Here's the drawing with two shaded views (mm, measured from the low corner). I have some questions. A direction names the side the tool comes from. Coordinates: 2 decimals unless noted, no trailing zeros. Write each loop counter-clockwise with the first axis right and the second up, starting at its lowest first coordinate (ties: lowest second). Pieces come first, ordered by that corner, then holes. Notation, with made-up numbers: (72, 25.5) -> (122, 25.5) arc R14 ccw to (122, 30.5) -> close; hole circle Ø1 at (-10, -8). An arc over 180 degrees is marked (long way). Use one line per item in the form item = value.
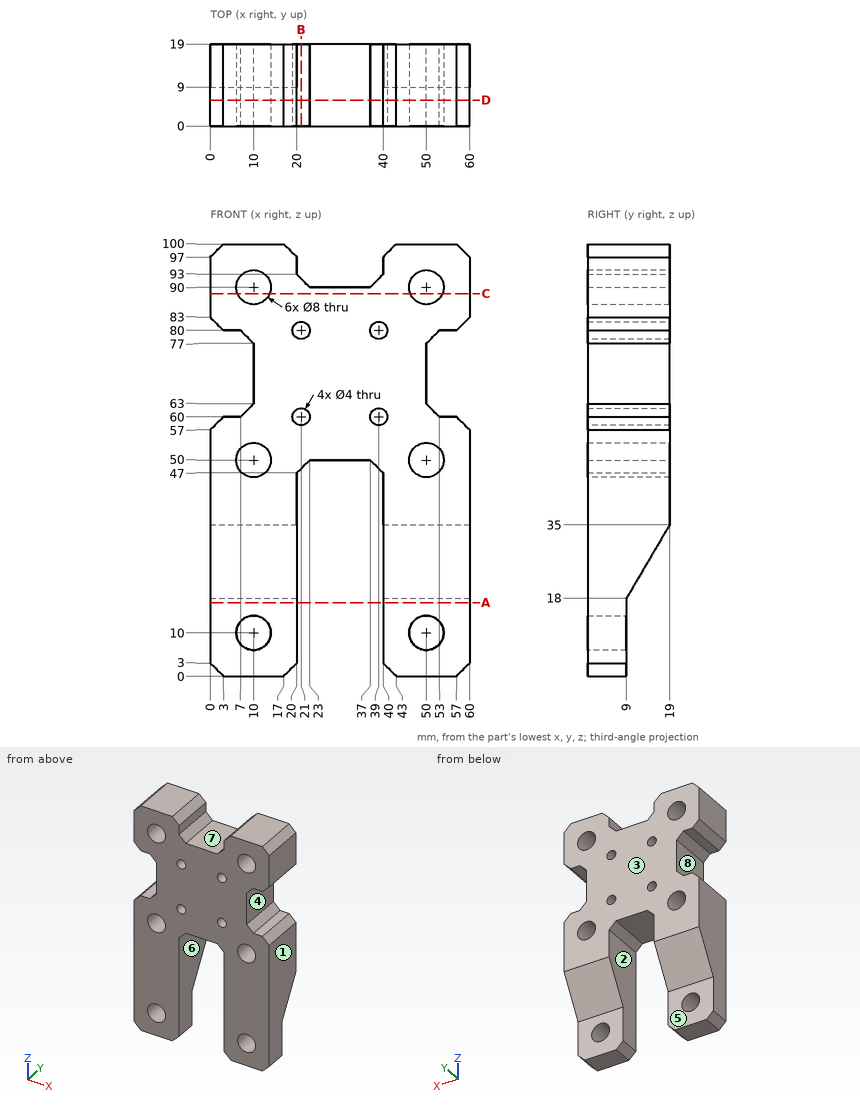
Q1. Suppose I cut it at A-A (z = 17). Write out the boundary of the cut face in (x, y), then the cut area to 3 significant figures.
Return value:
outline = (0, 0) -> (20, 0) -> (20, 9) -> (0, 9) -> close; (40, 0) -> (60, 0) -> (60, 9) -> (40, 9) -> close
area = 360 mm2
Q2. Suppose I cut it at B-B (x = 21). Write out the boundary of the cut face in (y, z).
Return value:
outline = (0, 48) -> (19, 48) -> (19, 58) -> (0, 58) -> close; (0, 62) -> (19, 62) -> (19, 78) -> (0, 78) -> close; (0, 82) -> (19, 82) -> (19, 92) -> (0, 92) -> close
Q3. If I drill on line 1 (X direction, y = 1.25, z = 31); line 2 (X direction, y = 2.25, z = 10); line 3 (X direction, y = 6.25, z = 86.5), over which ranges is the centre line in solid material (lowest first)? Write a range as from..to.
Return value:
line_1 = 0..20, 40..60
line_2 = 0..6, 14..20, 40..46, 54..60
line_3 = 0..8.06, 11.94..48.06, 51.94..60
Q4. Will these pins go through, and if not, where does the flat tip stop? pin 1 (8 mm diameter, centred on x = 37.5, z = 51, fed in from -Y); pin 2 (4 mm diameter, centred on x = 20, y = 5.5, fed in from -Z); pin 3 (11 mm diameter, centred on y = 9.5, z = 73, fed in from -X); pin 4 (5.5 mm diameter, centred on x = 8, z = 7, fed in from +Y).
Return value:
pin_1 = 0
pin_2 = 1
pin_3 = 8.5
pin_4 = 9
Q5. For the marked faces 4, 5, 6, 7 and 8, which set-ups out of +Z, -Z, +X, -X, +Y, -Y let a thin tool reach every point of the face, with its end or its side?
Return value:
face_4 = +X, +Y, -Y
face_5 = -Z, +X, -X, +Y
face_6 = -Z, +Y, -Y
face_7 = +Z, +Y, -Y
face_8 = -X, +Y, -Y
Q6. Suppose I cut it at D-D (y = 6). Give the number of separate pieces and of enclosed holes in the cut face, then the cut area to 3 significant figures.
Return value:
separate_pieces = 1
enclosed_holes = 10
area = 4,030 mm2
Q7. Suppose I cut it at C-C (z = 88.5). Write out the boundary of the cut face in (x, y).
Return value:
outline = (0, 0) -> (6.29, 0) -> (6.29, 19) -> (0, 19) -> close; (13.71, 0) -> (46.29, 0) -> (46.29, 19) -> (13.71, 19) -> close; (53.71, 0) -> (60, 0) -> (60, 19) -> (53.71, 19) -> close
Q8. Thinking about a two-plate mould opening in X: for the marked faces 1, 2 and 3, which applies, released by +X, released by -X, zero draft, split by the parting line, or undercut?
Return value:
face_1 = released by +X
face_2 = undercut
face_3 = zero draft
